Design review of the part built by this model. Coordinates are the model's own, in mm. Coordinates: 2 decimals unless noted, no trailing zeros. Order: outer loops, then holes, each group sorted by start corner. A loop starts at its lowest first (then second) coordinate and runs counter-clockwise, first axis right, second up. Notation, with made-up numbers: (-17, -36) -> (-7, -36) arc R10 ccw to (-7, -29) -> close; hole circle Ø5 at (-1, 33.5). An arc over 180 degrees is marked (long way). Write item = value, one per line.
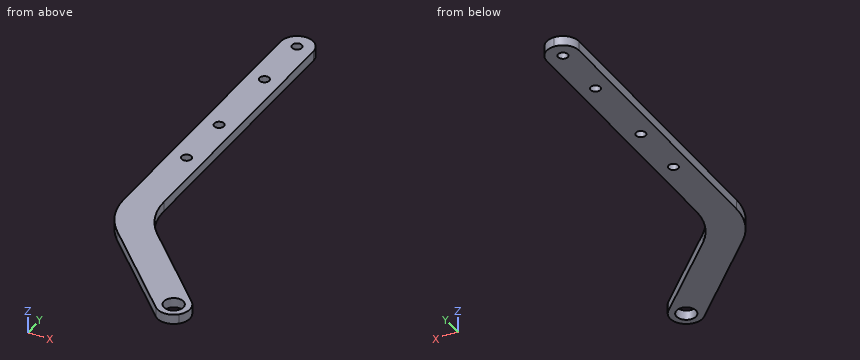
```python
from build123d import *

# Parameters (mm, degrees)
SKETCH_1_R      = 1.5
SKETCH_1_R_2    = 3
EXTRUDE_1_DEPTH = 3
FILLET_1_R      = 20
FILLET_2_R      = 5
FILLET_3_R      = 5


with BuildPart() as part:
    # 草图1 → 凸台-拉伸1 (new body)
    with BuildSketch(Plane.XY):
        Polygon((0, 0), (0, 100), (10, 100), (10, 4.142135624), (43.235357393, -29.093221769), (36.164289581, -36.164289581), align=None)
        with Locations((5, 34)):
            Circle(SKETCH_1_R, mode=Mode.SUBTRACT)
        with Locations((36.164289581, -29.093221769)):
            Circle(SKETCH_1_R_2, mode=Mode.SUBTRACT)
        with Locations((5, 52)):
            Circle(SKETCH_1_R, mode=Mode.SUBTRACT)
        with Locations((5, 77)):
            Circle(SKETCH_1_R, mode=Mode.SUBTRACT)
        with Locations((5, 95)):
            Circle(SKETCH_1_R, mode=Mode.SUBTRACT)
    extrude(amount=EXTRUDE_1_DEPTH)

    # 圆角1
    fillet_1_edges = [part.edges().sort_by_distance(p)[0] for p in [
        (0, 0, 1.5),
        (10, 4.142135624, 1.5),
    ]]
    fillet(fillet_1_edges, radius=FILLET_1_R)

    # 圆角2
    fillet_2_edges = [part.edges().sort_by_distance(p)[0] for p in [
        (36.164289581, -36.164289581, 1.5),
        (43.235357393, -29.093221769, 1.5),
    ]]
    fillet(fillet_2_edges, radius=FILLET_2_R - 0.0001)  # a hair under: the kernel refuses the full size

    # 圆角3
    fillet_3_edges = [part.edges().sort_by_distance(p)[0] for p in [
        (0, 100, 1.5),
        (10, 100, 1.5),
    ]]
    fillet(fillet_3_edges, radius=FILLET_3_R - 0.0001)  # a hair under: the kernel refuses the full size


solid = part.part
```
(1) We need section A-A (y = 52). Write out the cut boundary in (x, z).
Report:
outline = (0, 0) -> (3.5, 0) -> (3.5, 3) -> (0, 3) -> close; (6.5, 0) -> (10, 0) -> (10, 3) -> (6.5, 3) -> close
(2) We need section B-B (z = 2.35). Give the number of separate pieces and of enclosed holes in the cut face, and give its area (3 significant figures).
Report:
separate_pieces = 1
enclosed_holes = 5
area = 1,390 mm²
(3) Insertion check: pin 1 (0.9 mm diameter, centred on y = 48.5, z = 1, fed in from +X); pin 2 (2.5 mm diameter, centred on x = 5, y = 95, fed in from +Z). Each pin has a flat end and moves straight along its axis. Give the tip position at first contact, or say it passes through.
Report:
pin_1 = 10
pin_2 = through
(4) We need section C-C (x = 34.5). Write out the cut boundary in (y, z), and give its area (3 significant figures).
Report:
outline = (-33.81, 0) -> (-31.59, 0) -> (-31.59, 3) -> (-33.81, 3) -> close; (-26.6, 0) -> (-20.36, 0) -> (-20.36, 3) -> (-26.6, 3) -> close
area = 25.4 mm²
(5) For L1, parallel to X at y = 77, z = 1.6; L2, parallel to Y at x = 5, z = 1; L3, parallel to X at y = 92.5, z = 0.85, list the stretches that pass through material, from the lowest coordinate up.
Report:
L1 = 0 to 3.5, 6.5 to 10
L2 = -4.94 to 32.5, 35.5 to 50.5, 53.5 to 75.5, 78.5 to 93.5, 96.5 to 100
L3 = 0 to 10
(6) We need section D-D (x = 19). Write out the cut boundary in (y, z), and give its area (3 significant figures).
Report:
outline = (-19, 0) -> (-4.86, 0) -> (-4.86, 3) -> (-19, 3) -> close
area = 42.4 mm²
